Could you check a few things on this model? Use its own coordinates, in mm. Face numbers are marked on the shaded views. Coordinates: 2 decimals unless noted, no trailing zeros. Write each loop counter-clockwise with the first axis right and the second up, starting at its lowest first coordinate (ties: lowest second). Pieces come first, ordered by that corner, then holes.
Item 1: Thinking about a two-plate mould opening in Y: for the marked faces 1, 2, 3 and 4, which applies, +Y half, -Y half, draft (parallel to the pull), parting line (faces both ways), or undercut?
Item 2: If I drill on probe 1 along Y at (x, z) = (-10.5, 1.75); probe 2 along Z at (x, y) = (14.91, 40.4); probe 3 along X at (y, z) = (-27, 3.25), over which ranges is the centre line in solid material (lowest first)?
Item 3: For P1, Ø2, axis at y = 31.5, z = 8.5, coming from the +X side; P2, Ø4.5, axis at y = -14.5, z = 7.5, coming from the -X side, each with a flat end and sliding along its axis, tell me the tip position at first contact or that it passes through.
Item 4: I want a section at C-C on y = 36.5. Please give me the cut outline in (x, z).
Item 5: I want a section at B-B on x = 10. Please give me the cut outline in (y, z).
Item 6: I want a section at D-D on x = 16.5. Please give me the cut outline in (y, z), then the cut area to 3 significant figures.
from build123d import *

# Parameters (mm, degrees)
F1_DEPTH = 15
F2_SIZE  = 3
F3_R     = 5
F4_R     = 2.75
F5_DEPTH = 150


with BuildPart() as f1:
    # F0 (on Top) → F1 (new body)
    with BuildSketch(Plane.XY):
        Polygon((0, 37.5), (9, 37.5), (20, 37.5), (20, 42.5), (-20, 42.5), (-20, 37.5), (-9, 37.5), align=None)
        Polygon((9, -37.5), (9, 37.5), (0, 37.5), (-9, 37.5), (-9, -37.5), (0, -37.5), align=None)
        Polygon((20, -37.5), (9, -37.5), (0, -37.5), (-9, -37.5), (-20, -37.5), (-20, -42.5), (20, -42.5), align=None)
    extrude(amount=F1_DEPTH)

    # F2
    f2_edges = [f1.edges().sort_by_distance(p)[0] for p in [
        (9, 0, 0),
        (-9, 0, 0),
        (-9, 0, 15),
        (9, 0, 15),
    ]]
    chamfer(f2_edges, length=F2_SIZE)

    # F3
    f3_edges = [f1.edges().sort_by_distance(p)[0] for p in [
        (20, -40, 15),
        (-20, -40, 0),
        (-20, -40, 15),
        (20, -40, 0),
        (-20, 40, 15),
        (-20, 40, 0),
        (20, 40, 0),
        (20, 40, 15),
    ]]
    fillet(f3_edges, radius=F3_R)

    # F4 (on face) → F5 (cut)
    with BuildSketch(Plane(origin=(0, 42.5, 0), x_dir=(-1, 0, 0), z_dir=(0, 1, 0))):
        with BuildLine():
            ThreePointArc((17.66, 7.5), (14.91, 10.25), (12.16, 7.5))
            ThreePointArc((12.16, 7.5), (14.91, 4.75), (17.66, 7.5))
        make_face()
        with Locations((-14.91, 7.5)):
            Circle(F4_R)
    extrude(amount=-F5_DEPTH, mode=Mode.SUBTRACT)


solid = f1.part
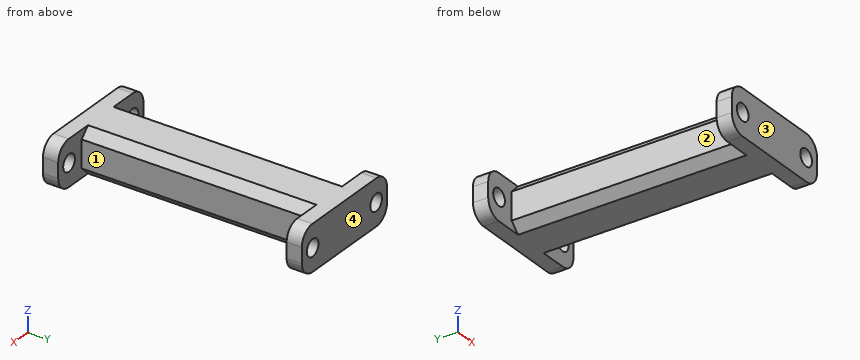
Response values:
1. face 1: undercut
1. face 2: undercut
1. face 3: -Y half
1. face 4: +Y half
2. probe 1: y = -42.5 to -37.5, 37.5 to 42.5
2. probe 2: z = 0 to 4.75, 10.25 to 15
2. probe 3: x = -9 to 9
3. P1: stops at x = 9
3. P2: stops at x = -9
4. outline: (-9, 3) - (-6, 0) - (6, 0) - (9, 3) - (9, 12) - (6, 15) - (-6, 15) - (-9, 12) - close
5. outline: (-42.5, 0) - (-37.5, 0) - (-37.5, 15) - (-42.5, 15) - close; (37.5, 0) - (42.5, 0) - (42.5, 15) - (37.5, 15) - close
6. outline: (-42.5, 0.23) - (-37.5, 0.23) - (-37.5, 5.26) - (-42.5, 5.26) - close; (-42.5, 9.74) - (-37.5, 9.74) - (-37.5, 14.77) - (-42.5, 14.77) - close; (37.5, 0.23) - (42.5, 0.23) - (42.5, 5.26) - (37.5, 5.26) - close; (37.5, 9.74) - (42.5, 9.74) - (42.5, 14.77) - (37.5, 14.77) - close
6. area: 101 mm2
